Study the drawing (mm; zero at the part's minimum x, y, z) and answer. Coordinates: 2 decimals unless noted, no trailing zeros. Loops run counter-clockwise (first coordinate to the right, second up) from the corner with the lowest first, then second, coordinate; pieces in that order, holes last. Notation, with made-up numbers: (-34, 46.25) - (-18, 46.25) arc R22 cw to (-18, 68.25) - close; hole circle Ø2 at (71, 55.25). An arc over 180 degrees is marked (long way). Put each result on its own line as item: value.
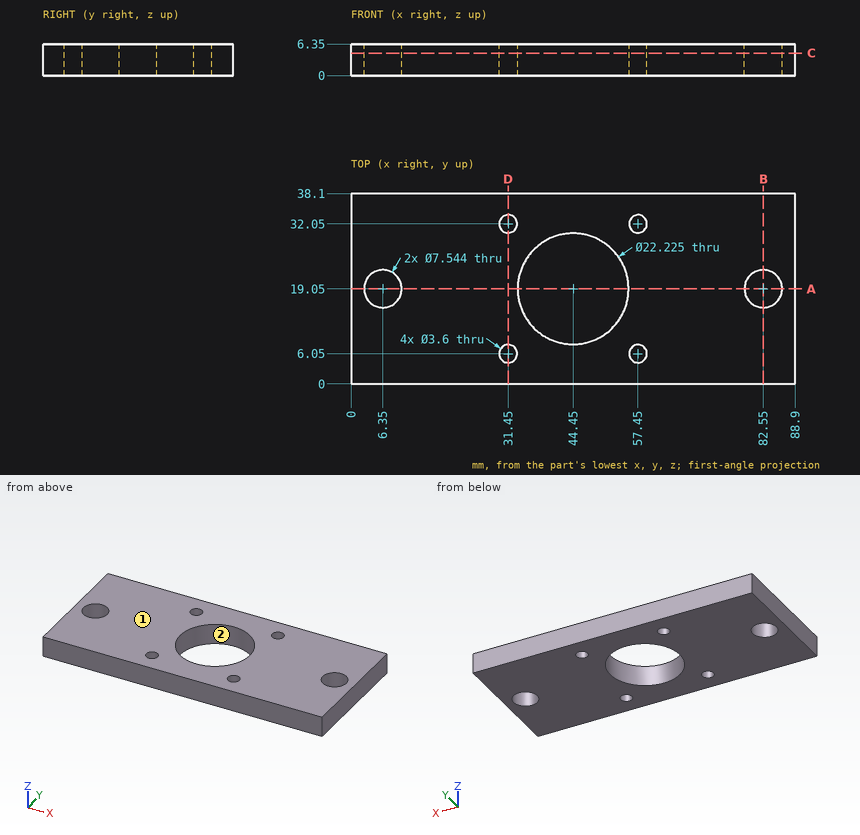
1) Straight lines are drawn through the part: L1, parallel to Y at x = 57.45, z = 3.25; L2, parallel to X at y = 32.05, z = 3.25; L3, parallel to X at y = 19, z = 4.5. For each, find the intervals that lie inside material, in ascending order. Write a range as [from, to].
Found:
L1: y = [0, 4.25], [7.85, 30.25], [33.85, 38.1]
L2: x = [0, 29.65], [33.25, 55.65], [59.25, 88.9]
L3: x = [0, 2.58], [10.12, 33.34], [55.56, 78.78], [86.32, 88.9]
2) The part is cut by section A-A (y = 19.05). Give the vertices of the cut face in (x, z), and give its area (3 significant figures).
Found:
outline: (0, 0) - (2.58, 0) - (2.58, 6.35) - (0, 6.35) - close; (10.12, 0) - (33.34, 0) - (33.34, 6.35) - (10.12, 6.35) - close; (55.56, 0) - (78.78, 0) - (78.78, 6.35) - (55.56, 6.35) - close; (86.32, 0) - (88.9, 0) - (88.9, 6.35) - (86.32, 6.35) - close
area: 328 mm^2
3) For a pull along X with two mould halves and no side action, classify the marked faces 1 and 2 as pulls with the +X half, pulls with the -X half, needs draft (parallel to the pull), parting line crosses it, or undercut.
Found:
face 1: needs draft
face 2: undercut
4) The part is cut by section D-D (x = 31.45). Give the vertices of the cut face in (y, z), and give its area (3 significant figures).
Found:
outline: (0, 0) - (4.25, 0) - (4.25, 6.35) - (0, 6.35) - close; (7.85, 0) - (30.25, 0) - (30.25, 6.35) - (7.85, 6.35) - close; (33.85, 0) - (38.1, 0) - (38.1, 6.35) - (33.85, 6.35) - close
area: 196 mm^2
5) The part is cut by section B-B (x = 82.55). Give the vertices of the cut face in (y, z).
Found:
outline: (0, 0) - (15.28, 0) - (15.28, 6.35) - (0, 6.35) - close; (22.82, 0) - (38.1, 0) - (38.1, 6.35) - (22.82, 6.35) - close
6) The part is cut by section C-C (z = 4.5). State how many separate pieces and enclosed holes the cut face has, and give its area (3 significant figures).
Found:
separate pieces: 1
enclosed holes: 7
area: 2,870 mm^2
